```python
from build123d import *

# Parameters (mm, degrees)
T_LE_DE_BASE_PLI_E1_DEPTH     = 60
ENL_V_MAT_EXTRU_1_REACH       = 84.492
ESQUISSE7_W                   = 24.5
ESQUISSE7_H                   = 45.3
ENL_V_MAT_EXTRU_2_REACH       = 84.492
ESQUISSE8_R                   = 1.3
ENL_V_MAT_EXTRU_3_REACH       = 81.889
ESQUISSE9_R                   = 2.25
CONG_1_R                      = 3
CONG_2_R                      = 5
ENL_V_MAT_EXTRU_4_OUTLINE_W   = 9
ENL_V_MAT_EXTRU_4_OUTLINE_H   = 60
ENL_V_MAT_EXTRU_4_DEPTH       = 28.15
ENL_V_START                   = -2.5
ENL_V_MAT_EXTRU_4_2_OUTLINE_W = 2.5
ENL_V_MAT_EXTRU_4_2_OUTLINE_H = 60
ENL_V_MAT_EXTRU_4_2_DEPTH     = 2.5
ENL_V_START_2                 = -4.85
ENL_V_MAT_EXTRU_4_3_OUTLINE_R = 2.25
ENL_V_MAT_EXTRU_4_3_OUTLINE_W = 4.160785036
ENL_V_MAT_EXTRU_4_3_OUTLINE_H = 60
ENL_V_MAT_EXTRU_4_3_DEPTH     = 4.85
ENL_V_MAT_EXTRU_4_4_OUTLINE_W = 2.5
ENL_V_MAT_EXTRU_4_4_OUTLINE_H = 60
ENL_V_MAT_EXTRU_4_4_DEPTH     = 2.35


# Read off the part's stored shape, not the designer's step: Tôle de base pliée1, Enlèv. mat.-Extru.4
with BuildPart() as part:
    # Tôle de base pliée1 outline → Tôle de base pliée1 (new body)
    with BuildSketch(Plane.XY):
        with BuildLine():
            Line((7.85, 28.15), (46, 28.15))
            Line((46, 28.15), (46, 33))
            Line((46, 33), (7.85, 33))
            ThreePointArc((7.85, 33), (2.299211768, 30.700788232), (0, 25.15))
            Line((0, 25.15), (0, 0))
            Line((0, 0), (4.85, 0))
            Line((4.85, 0), (4.85, 25.15))
            ThreePointArc((4.85, 25.15), (5.728679656, 27.271320344), (7.85, 28.15))
        make_face()
    extrude(amount=T_LE_DE_BASE_PLI_E1_DEPTH)

    # Esquisse7 → Enlèv. mat.-Extru.1 (cut, up to next)
    with BuildSketch(Plane(origin=(0, 33, 0), x_dir=(1, 0, 0), z_dir=(0, 1, 0)), mode=Mode.PRIVATE) as enl_v_mat_extru_1_sk1:
        with Locations((26.75, -30)):
            Rectangle(ESQUISSE7_W, ESQUISSE7_H)
    enl_v_mat_extru_1_tool1 = extrude(enl_v_mat_extru_1_sk1.sketch, amount=-ENL_V_MAT_EXTRU_1_REACH, mode=Mode.PRIVATE) & part.part
    add(enl_v_mat_extru_1_tool1.solids().sort_by_distance((26.75, 33, 30))[0], mode=Mode.SUBTRACT)

    # Esquisse8 → Enlèv. mat.-Extru.2 (cut, up to next)
    with BuildSketch(Plane(origin=(0, 33, 0), x_dir=(1, 0, 0), z_dir=(0, 1, 0)), mode=Mode.PRIVATE) as enl_v_mat_extru_2_sk1:
        with Locations(Location((18.25, -55.3, 0), (0, 0, 270))):
            Circle(ESQUISSE8_R)
    enl_v_mat_extru_2_tool1 = extrude(enl_v_mat_extru_2_sk1.sketch, amount=-ENL_V_MAT_EXTRU_2_REACH, mode=Mode.PRIVATE) & part.part
    # Esquisse8 → Enlèv. mat.-Extru.2 (cut, up to next)
    with BuildSketch(Plane(origin=(0, 33, 0), x_dir=(1, 0, 0), z_dir=(0, 1, 0)), mode=Mode.PRIVATE) as enl_v_mat_extru_2_sk2:
        with Locations(Location((35.25, -55.3, 0), (0, 0, 270))):
            Circle(ESQUISSE8_R)
    enl_v_mat_extru_2_tool2 = extrude(enl_v_mat_extru_2_sk2.sketch, amount=-ENL_V_MAT_EXTRU_2_REACH, mode=Mode.PRIVATE) & part.part
    # Esquisse8 → Enlèv. mat.-Extru.2 (cut, up to next)
    with BuildSketch(Plane(origin=(0, 33, 0), x_dir=(1, 0, 0), z_dir=(0, 1, 0)), mode=Mode.PRIVATE) as enl_v_mat_extru_2_sk3:
        with Locations(Location((41.3, -15, 0), (0, 0, 270))):
            Circle(ESQUISSE8_R)
    enl_v_mat_extru_2_tool3 = extrude(enl_v_mat_extru_2_sk3.sketch, amount=-ENL_V_MAT_EXTRU_2_REACH, mode=Mode.PRIVATE) & part.part
    # Esquisse8 → Enlèv. mat.-Extru.2 (cut, up to next)
    with BuildSketch(Plane(origin=(0, 33, 0), x_dir=(1, 0, 0), z_dir=(0, 1, 0)), mode=Mode.PRIVATE) as enl_v_mat_extru_2_sk4:
        with Locations(Location((12.2, -15, 0), (0, 0, 270))):
            Circle(ESQUISSE8_R)
    enl_v_mat_extru_2_tool4 = extrude(enl_v_mat_extru_2_sk4.sketch, amount=-ENL_V_MAT_EXTRU_2_REACH, mode=Mode.PRIVATE) & part.part
    add(enl_v_mat_extru_2_tool1.solids().sort_by_distance((18.25, 33, 55.3))[0], mode=Mode.SUBTRACT)
    add(enl_v_mat_extru_2_tool2.solids().sort_by_distance((35.25, 33, 55.3))[0], mode=Mode.SUBTRACT)
    add(enl_v_mat_extru_2_tool3.solids().sort_by_distance((41.3, 33, 15))[0], mode=Mode.SUBTRACT)
    add(enl_v_mat_extru_2_tool4.solids().sort_by_distance((12.2, 33, 15))[0], mode=Mode.SUBTRACT)

    # Esquisse9 → Enlèv. mat.-Extru.3 (cut, up to next)
    with BuildSketch(Plane(origin=(4.85, 0, 0), x_dir=(0, 0, -1), z_dir=(1, 0, 0)), mode=Mode.PRIVATE) as enl_v_mat_extru_3_sk1:
        with Locations((-4.5, 5)):
            Circle(ESQUISSE9_R)
    enl_v_mat_extru_3_tool1 = extrude(enl_v_mat_extru_3_sk1.sketch, amount=-ENL_V_MAT_EXTRU_3_REACH, mode=Mode.PRIVATE) & part.part
    # Esquisse9 → Enlèv. mat.-Extru.3 (cut, up to next)
    with BuildSketch(Plane(origin=(4.85, 0, 0), x_dir=(0, 0, -1), z_dir=(1, 0, 0)), mode=Mode.PRIVATE) as enl_v_mat_extru_3_sk2:
        with Locations(Location((-4.5, 21, 0), (0, 0, 180))):
            Circle(ESQUISSE9_R)
    enl_v_mat_extru_3_tool2 = extrude(enl_v_mat_extru_3_sk2.sketch, amount=-ENL_V_MAT_EXTRU_3_REACH, mode=Mode.PRIVATE) & part.part
    # Esquisse9 → Enlèv. mat.-Extru.3 (cut, up to next)
    with BuildSketch(Plane(origin=(4.85, 0, 0), x_dir=(0, 0, -1), z_dir=(1, 0, 0)), mode=Mode.PRIVATE) as enl_v_mat_extru_3_sk3:
        with Locations((-55.5, 21)):
            Circle(ESQUISSE9_R)
    enl_v_mat_extru_3_tool3 = extrude(enl_v_mat_extru_3_sk3.sketch, amount=-ENL_V_MAT_EXTRU_3_REACH, mode=Mode.PRIVATE) & part.part
    # Esquisse9 → Enlèv. mat.-Extru.3 (cut, up to next)
    with BuildSketch(Plane(origin=(4.85, 0, 0), x_dir=(0, 0, -1), z_dir=(1, 0, 0)), mode=Mode.PRIVATE) as enl_v_mat_extru_3_sk4:
        with Locations(Location((-55.5, 5, 0), (0, 0, 180))):
            Circle(ESQUISSE9_R)
    enl_v_mat_extru_3_tool4 = extrude(enl_v_mat_extru_3_sk4.sketch, amount=-ENL_V_MAT_EXTRU_3_REACH, mode=Mode.PRIVATE) & part.part
    add(enl_v_mat_extru_3_tool1.solids().sort_by_distance((4.85, 5, 4.5))[0], mode=Mode.SUBTRACT)
    add(enl_v_mat_extru_3_tool2.solids().sort_by_distance((4.85, 21, 4.5))[0], mode=Mode.SUBTRACT)
    add(enl_v_mat_extru_3_tool3.solids().sort_by_distance((4.85, 21, 55.5))[0], mode=Mode.SUBTRACT)
    add(enl_v_mat_extru_3_tool4.solids().sort_by_distance((4.85, 5, 55.5))[0], mode=Mode.SUBTRACT)

    # Congé1
    cong_1_edges = [part.edges().sort_by_distance(p)[0] for p in [
        (14.5, 30.575, 52.65),
        (14.5, 30.575, 7.35),
        (39, 30.575, 7.35),
        (39, 30.575, 52.65),
    ]]
    fillet(cong_1_edges, radius=CONG_1_R)

    # Congé2
    cong_2_edges = [part.edges().sort_by_distance(p)[0] for p in [
        (2.425, 0, 60),
        (46, 30.575, 60),
        (2.425, 0, 0),
        (46, 30.575, 0),
    ]]
    fillet(cong_2_edges, radius=CONG_2_R)

    # Enlèv. mat.-Extru.4 outline → Enlèv. mat.-Extru.4 (cut)
    with BuildSketch(Plane.XZ.offset(-28.15)):
        with Locations((4.5, 30)):
            Rectangle(ENL_V_MAT_EXTRU_4_OUTLINE_W, ENL_V_MAT_EXTRU_4_OUTLINE_H)
    extrude(amount=ENL_V_MAT_EXTRU_4_DEPTH, mode=Mode.SUBTRACT)

    # Enl_v. mat.-Extru.4 2 outline → Enl_v. mat.-Extru.4 2 (cut)
    with BuildSketch(Plane.XZ.offset(-28.15).offset(ENL_V_START)):
        with Locations((3.589214964, 30)):
            Rectangle(ENL_V_MAT_EXTRU_4_2_OUTLINE_W, ENL_V_MAT_EXTRU_4_2_OUTLINE_H)
    extrude(amount=ENL_V_MAT_EXTRU_4_2_DEPTH, mode=Mode.SUBTRACT)

    # Enl_v. mat.-Extru.4 3 outline → Enl_v. mat.-Extru.4 3 (add)
    # profile 1 of 2: a face of its own
    with BuildSketch(Plane.XZ.offset(-28.15).offset(ENL_V_START_2)):
        with BuildLine():
            ThreePointArc((-25.821570073, 5), (-24.357103979, 1.464466094), (-20.821570073, 0))
            Line((-20.821570073, 0), (2.339214964, 0))
            Line((2.339214964, 0), (2.339214964, 60))
            Line((2.339214964, 60), (-20.821570073, 60))
            ThreePointArc((-20.821570073, 60), (-24.357103979, 58.535533906), (-25.821570073, 55))
            Line((-25.821570073, 55), (-25.821570073, 5))
        make_face()
        with Locations((-20.821570073, 4.5)):
            Circle(ENL_V_MAT_EXTRU_4_3_OUTLINE_R, mode=Mode.SUBTRACT)
        with Locations((-4.821570073, 4.5)):
            Circle(ENL_V_MAT_EXTRU_4_3_OUTLINE_R, mode=Mode.SUBTRACT)
        with Locations((-20.821570073, 55.5)):
            Circle(ENL_V_MAT_EXTRU_4_3_OUTLINE_R, mode=Mode.SUBTRACT)
        with Locations((-4.821570073, 55.5)):
            Circle(ENL_V_MAT_EXTRU_4_3_OUTLINE_R, mode=Mode.SUBTRACT)
    # profile 2 of 2: a face of its own
    with BuildSketch(Plane.XZ.offset(-28.15).offset(ENL_V_START_2)):
        with Locations((6.919607482, 30)):
            Rectangle(ENL_V_MAT_EXTRU_4_3_OUTLINE_W, ENL_V_MAT_EXTRU_4_3_OUTLINE_H)
    extrude(amount=ENL_V_MAT_EXTRU_4_3_DEPTH)

    # Enl_v. mat.-Extru.4 4 outline → Enl_v. mat.-Extru.4 4 (add)
    with BuildSketch(Plane.XZ.offset(-28.15).offset(ENL_V_START_2)):
        with Locations((3.589214964, 30)):
            Rectangle(ENL_V_MAT_EXTRU_4_4_OUTLINE_W, ENL_V_MAT_EXTRU_4_4_OUTLINE_H)
    extrude(amount=ENL_V_MAT_EXTRU_4_4_DEPTH)


solid = part.part
```
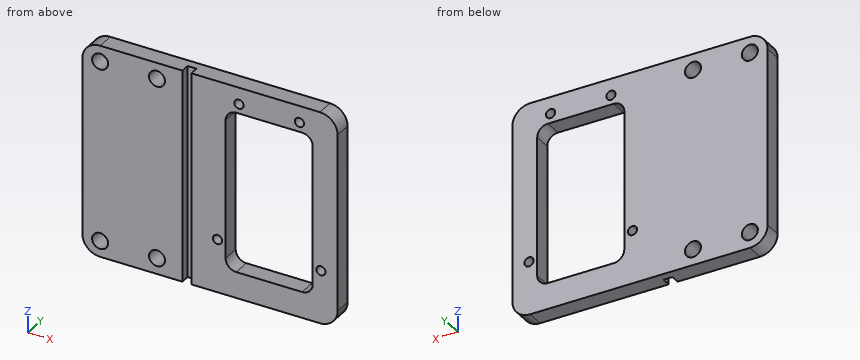
Input: part model. Units: mm. Frame: model coordinates. Give positions to 0.01 mm unless a question says otherwise; leave off trailing zeros. Loops run counter-clockwise (first coordinate to the right, second up) from the corner with the lowest first, then second, coordinate; pieces in that order, holes last. Notation, with made-up numbers: M 35,79.5 L 87,79.5 A25 cw 87,96.5 Z; hole C -9.5,5.25 d11. An arc over 180 degrees is marked long. Answer as CSV lines item,"result". Start each with the question number.
1. Line query: L1, parallel to X at y = 29.8, z = 31; L2, parallel to X at y = 31.75, z = 55.3; L3, parallel to Z at x = 32, y = 28.9. Output: solid intervals per line, ascending.
2. Section A-A on y = 29.85. State how many separate pieces and enclosed holes the cut face has, plus the area to 3 significant figures.
3. Section B-B on x = 29. Return loops of the section in (y, z).
4. Section C-C on z = 30. Return loops of the section in (x, y).
5. Section D-D on z = 15. Return loops of the section in (x, y), plus the area to 3 significant figures.
6. Pin query (flat end, axial travel): P1, Ø3.5, axis at x = -20.82, z = 55.5, coming from the +Y side; P2, Ø0.8, axis at x = 3.5, z = 18, coming from the -Y side. Return the tip coordinate at first contact, or that it passes through.
Computed values:
1,L1,"x = -25.82 to 2.34, 4.84 to 14.5, 39 to 46"
1,L2,"x = -25.81 to -23.06, -18.58 to -7.06, -2.58 to 16.95, 19.55 to 33.95, 36.55 to 45.99"
1,L3,"z = 0 to 7.35, 52.65 to 60"
2,separate pieces,"2"
2,enclosed holes,"9"
2,area,"2,950 mm²"
3,outline,"M 28.15,0 L 33,0 L 33,7.35 L 28.15,7.35 Z; M 28.15,52.65 L 33,52.65 L 33,60 L 28.15,60 Z"
4,outline,"M -25.82,28.15 L 2.34,28.15 L 2.34,30.65 L 4.84,30.65 L 4.84,28.15 L 14.5,28.15 L 14.5,33 L -25.82,33 Z; M 39,28.15 L 46,28.15 L 46,33 L 39,33 Z"
5,outline,"M -25.82,28.15 L 2.34,28.15 L 2.34,30.65 L 4.84,30.65 L 4.84,28.15 L 10.9,28.15 L 10.9,33 L -25.82,33 Z; M 13.5,28.15 L 14.5,28.15 L 14.5,33 L 13.5,33 Z; M 39,28.15 L 40,28.15 L 40,33 L 39,33 Z; M 42.6,28.15 L 46,28.15 L 46,33 L 42.6,33 Z"
5,area,"198 mm²"
6,P1,"passes through"
6,P2,"stops at y = 30.65"
